```python
from build123d import *

# Parameters (mm, degrees)
BASEFLANGE_W                 = 1000
BASEFLANGE_H                 = 50
BASEFLANGE1_DEPTH            = 2
EDGE_FLANGE2_STRIP_W         = 10
EDGE_FLANGE2_STRIP_H         = 2
EDGE_FLANGE2_STRIP_CUT_DEPTH = 1000
EDGE_FLANGE2_DEPTH           = 1000
SKETCH12_R                   = 2.1
F_4_2MM_HOLE_DEPTH           = 10
SLOT_1_DEPTH                 = 10
LEFT_EDGE_STRIP_W            = 10
LEFT_EDGE_STRIP_H            = 2
LEFT_EDGE_STRIP_CUT_DEPTH    = 47
LEFT_EDGE_DEPTH              = 47
CUT_EXTRUDE1_DEPTH           = 1002.561281201
CUT_EXTRUDE1_DEPTH_BACK      = 1002.561281201
SKETCH19_R                   = 2.1
RIGHT_EDGE_STRIP_W           = 10
RIGHT_EDGE_STRIP_H           = 2
RIGHT_EDGE_STRIP_CUT_DEPTH   = 47
RIGHT_EDGE_DEPTH             = 47
CUT_EXTRUDE2_START           = -10
SKETCH25_R                   = 2.1
CUT_EXTRUDE2_DEPTH           = 10


# Sheet-metal steps are written as plain solids
with BuildPart() as part:
    # BaseFlange → BaseFlange1 (new body)
    with BuildSketch(Plane.XY):
        Rectangle(BASEFLANGE_W, BASEFLANGE_H)
    extrude(amount=BASEFLANGE1_DEPTH)

    # Edge-Flange2 strip (across the edge) → Edge-Flange2 strip cut (cut)
    with BuildSketch(Plane(origin=(-500, -25, 2), x_dir=(0, 1, 0), z_dir=(1, 0, 0))):
        with Locations((-2, -1)):
            Rectangle(EDGE_FLANGE2_STRIP_W, EDGE_FLANGE2_STRIP_H)
    extrude(amount=EDGE_FLANGE2_STRIP_CUT_DEPTH, mode=Mode.SUBTRACT)

    # Edge-Flange2 section (across the edge) → Edge-Flange2 (add)
    with BuildSketch(Plane(origin=(-500, -25, 2), x_dir=(0, 1, 0), z_dir=(1, 0, 0))):
        with BuildLine():
            Line((0, 1), (0, 48))
            Line((0, 48), (2, 48))
            Line((2, 48), (2, 1))
            ThreePointArc((2, 1), (2.292893219, 0.292893219), (3, 0))
            Line((3, 0), (3, -2))
            ThreePointArc((3, -2), (0.878679656, -1.121320344), (0, 1))
        make_face()
    extrude(amount=EDGE_FLANGE2_DEPTH)

    # Sketch12 → 4.2mm Hole (cut)
    with BuildSketch(Plane(origin=(0, -23, 0), x_dir=(1, 0, 0), z_dir=(0, 1, 0))):
        with Locations(Location((460, -25, 0), (0, 0, 270))):
            Circle(SKETCH12_R)
    extrude(amount=-F_4_2MM_HOLE_DEPTH, mode=Mode.SUBTRACT)

    # slot1 → Slot 1 (cut)
    with BuildSketch(Plane.XY.offset(2)):
        with BuildLine():
            Line((468.5, 4.25), (481.5, 4.25))
            ThreePointArc((481.5, 4.25), (485.75, 0), (481.5, -4.25))
            Line((481.5, -4.25), (468.5, -4.25))
            ThreePointArc((468.5, -4.25), (464.25, 0), (468.5, 4.25))
        make_face()
    slot_1 = extrude(amount=-SLOT_1_DEPTH, mode=Mode.SUBTRACT)

    # Slot Pattern: Slot 1 at 1 more place
    with Locations((-950, 0, 0)):
        add(slot_1, mode=Mode.SUBTRACT)

    # Left Edge strip (across the edge) → Left Edge strip cut (cut)
    with BuildSketch(Plane(origin=(-500, 25, 2), x_dir=(1, 0, 0), z_dir=(0, -1, 0))):
        with Locations((-2, -1)):
            Rectangle(LEFT_EDGE_STRIP_W, LEFT_EDGE_STRIP_H)
    extrude(amount=LEFT_EDGE_STRIP_CUT_DEPTH, mode=Mode.SUBTRACT)

    # Left Edge section (across the edge) → Left Edge (add)
    with BuildSketch(Plane(origin=(-500, 25, 2), x_dir=(1, 0, 0), z_dir=(0, -1, 0))):
        with BuildLine():
            Line((0, 1), (0, 48))
            Line((0, 48), (2, 48))
            Line((2, 48), (2, 1))
            ThreePointArc((2, 1), (2.292893219, 0.292893219), (3, 0))
            Line((3, 0), (3, -2))
            ThreePointArc((3, -2), (0.878679656, -1.121320344), (0, 1))
        make_face()
    extrude(amount=LEFT_EDGE_DEPTH)

    # Sketch19 → Cut-Extrude1 (cut, two sides: drawn at the far end of the back side and taken through both)
    with BuildSketch(Plane.ZY.offset(500).offset(-CUT_EXTRUDE1_DEPTH_BACK)):
        with Locations((25, 0)):
            Circle(SKETCH19_R)
    extrude(amount=CUT_EXTRUDE1_DEPTH + CUT_EXTRUDE1_DEPTH_BACK, mode=Mode.SUBTRACT)

    # Right Edge strip (across the edge) → Right Edge strip cut (cut)
    with BuildSketch(Plane(origin=(500, -22, 2), x_dir=(-1, 0, 0), z_dir=(0, 1, 0))):
        with Locations((-2, -1)):
            Rectangle(RIGHT_EDGE_STRIP_W, RIGHT_EDGE_STRIP_H)
    extrude(amount=RIGHT_EDGE_STRIP_CUT_DEPTH, mode=Mode.SUBTRACT)

    # Right Edge section (across the edge) → Right Edge (add)
    with BuildSketch(Plane(origin=(500, -22, 2), x_dir=(-1, 0, 0), z_dir=(0, 1, 0))):
        with BuildLine():
            Line((0, 1), (0, 48))
            Line((0, 48), (2, 48))
            Line((2, 48), (2, 1))
            ThreePointArc((2, 1), (2.292893219, 0.292893219), (3, 0))
            Line((3, 0), (3, -2))
            ThreePointArc((3, -2), (0.878679656, -1.121320344), (0, 1))
        make_face()
    extrude(amount=RIGHT_EDGE_DEPTH)

    # Sketch25 → Cut-Extrude2 (cut)
    with BuildSketch(Plane(origin=(500, 0, 0), x_dir=(0, 0, -1), z_dir=(1, 0, 0)).offset(CUT_EXTRUDE2_START)):
        with Locations(Location((-25, 0, 0), (0, 0, 180))):
            Circle(SKETCH25_R)
    extrude(amount=CUT_EXTRUDE2_DEPTH, mode=Mode.SUBTRACT)


solid = part.part
```
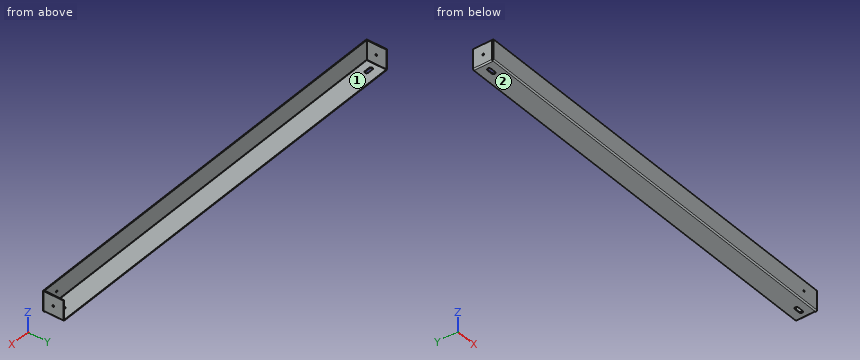
The listing builds one solid part. Answer for the finished solid, in the listing's coordinates (mm). Face numbers are marked on the shaded views. A direction names the side the tool comes from. Give positions to 0.01 mm unless a question says otherwise; leave off trailing zeros. Write each loop counter-clockwise with the first axis right and the second up, starting at its lowest first coordinate (ties: lowest second). Pieces come first, ordered by that corner, then holes. Notation, with made-up numbers: (-8, 7.5) -> (24, 7.5) arc R16 ccw to (24, 11.5) -> close; hole circle Ø7 at (25.5, -30.75). An arc over 180 degrees is marked (long way). Write item = value, one per line. Start each with the question number.
1) The part is cut by section A-A, the plane z = 41. Determine the outline of the cut face in (x, y), and give its area (3 significant figures).
2) The part is cut by section B-B, the plane x = -70. Determine the outline of the cut face in (y, z).
3) Which of the six approach directions +Z, -Z, +X, -X, +Y, -Y give full straight-line access (tool end or side, diameter ignored) to the marked faces 1 and 2?
4) Straight lines are drawn through the part: line 1 along Y through (x, z) = (-499, 25); line 2 along X through (y, z) = (12, 22.5); line 3 along Y through (x, z) = (274, 16). For each, find the intervals that lie inside material, in ascending order.
5) Each of these flat-tipped pins is pushed along its axis until it touches: pin 1 (1 mm diameter, centred on x = -473.5, z = 0.5, fed in from -Y); pin 2 (1.5 mm diameter, centred on x = 239.5, z = 27.5, fed in from +Y); pin 3 (1.6 mm diameter, centred on x = 472.5, z = 1, fed in from -Y); pin 4 (2.5 mm diameter, centred on y = 0, z = 25, fed in from -X). Where does it stop, or does it pass through?
Solutions:
q1.outline = (-500, -25) -> (500, -25) -> (500, -23) -> (-500, -23) -> close; (-500, -22) -> (-498, -22) -> (-498, 25) -> (-500, 25) -> close; (498, -22) -> (500, -22) -> (500, 25) -> (498, 25) -> close
q1.area = 2,190 mm²
q2.outline = (-25, 3) arc R3 ccw to (-22, 0) -> (25, 0) -> (25, 2) -> (-22, 2) arc R1 cw to (-23, 3) -> (-23, 50) -> (-25, 50) -> close
q3.face_1 = +Z, +Y
q3.face_2 = -Z, +X, -X, +Y, -Y
q4.line_1 = -25 to -23, -22 to -2.1, 2.1 to 25
q4.line_2 = -500 to -498, 498 to 500
q4.line_3 = -25 to -23
q5.pin_1 = -24.24
q5.pin_2 = -23
q5.pin_3 = -24.75
q5.pin_4 = through
